```python
from build123d import *

# Parameters (mm, degrees)
CBORE_FOR_M3_HEX_SOCKET_HEAD_CAP_SCREW1_D           = 3.4
CBORE_FOR_M3_HEX_SOCKET_HEAD_CAP_SCREW1_CBORE_D     = 6.5
CBORE_FOR_M3_HEX_SOCKET_HEAD_CAP_SCREW1_CBORE_DEPTH = 3.4
F_20_0MM_DOWEL_HOLE1_D                              = 20


# Read off the part's stored shape, not the designer's step: M30 Machine Threads Stud1
with BuildPart() as part:
    # Sketch1 → Revolve1 (revolve)
    with BuildSketch(Plane.XY, mode=Mode.PRIVATE) as revolve1_sk:
        Polygon((0, 0), (41, 0), (41, 16), (6, 16), (6, 26), (0, 26), align=None)
    revolve(revolve1_sk.sketch.rotate(Axis((0, 0, 0), (1, 0, 0)), 90), axis=Axis((0, 0, 0), (1, 0, 0)))

    # M30 Machine Threads Stud1 outline → M30 Machine Threads Stud1 (revolve, cut)
    with BuildSketch(Plane.YX):
        Polygon((16, 41), (13.079, 41), (15, 39.079), (15, 26), (16, 26), align=None)
    revolve(axis=Axis((0, 0, 0), (1, 0, 0)), mode=Mode.SUBTRACT)

    # CBORE for M3 Hex Socket Head Cap Screw1 (through all)
    with Locations(Plane.ZY):
        with Locations((-21, 0), (0, 21), (21, 0), (0, -21)):
            CounterBoreHole(CBORE_FOR_M3_HEX_SOCKET_HEAD_CAP_SCREW1_D / 2, CBORE_FOR_M3_HEX_SOCKET_HEAD_CAP_SCREW1_CBORE_D / 2, CBORE_FOR_M3_HEX_SOCKET_HEAD_CAP_SCREW1_CBORE_DEPTH)

    # Ø20.0mm Dowel Hole1 (through all)
    with Locations(Plane.ZY):
        with Locations((0, 0)):
            Hole(F_20_0MM_DOWEL_HOLE1_D / 2)

    # Sketch9 → Cut-Revolve1 (revolve, cut)
    with BuildSketch(Plane.XY, mode=Mode.PRIVATE) as cut_revolve1_sk:
        Polygon((30, 15), (28.5, 13.5), (26, 13.5), (26, 15), align=None)
    revolve(cut_revolve1_sk.sketch.rotate(Axis((0, 0, 0), (1, 0, 0)), 90), axis=Axis((0, 0, 0), (1, 0, 0)), mode=Mode.SUBTRACT)


solid = part.part
```
Geometry check sheet. Reference: the model listing, model coordinates, mm. A direction names the side the tool comes from. Round coordinates to 2 decimals unless told otherwise and drop trailing zeros. Loops run counter-clockwise (first coordinate to the right, second up) from the corner with the lowest first, then second, coordinate; pieces in that order, holes last. Notation, with made-up numbers: (79.5, 76.25) - (127.5, 76.25) arc R32 cw to (127.5, 111.25) - close; hole circle Ø1 at (51.5, 23). An arc over 180 degrees is marked (long way). Write each question's results on one line, items separated by ' | '. Start each with the question number.
Q1. Gauge pin test, flat ends, axial feed: P1, Ø2, axis at y = 4, z = -20, coming from the +X side; P2, Ø6, axis at x = 13.5, y = -2, coming from the +Z side; P3, Ø4, axis at y = 21, z = 0, coming from the -X side; P4, Ø2, axis at y = 0, z = 21, coming from the -X side. Record the tip position at first contact, or that the pin passes through.
Q2. Thickness scan on line 1 (Y direction, x = 4, z = 0); line 2 (Y direction, x = 1.6, z = 0); line 3 (Y direction, x = 21, z = 0). Record the ranges inside material, lowest first. Write a range as [from, to].
Q3. Cross-section at C-C on y = 0. State how many separate pieces and enclosed holes the cut face has, and give its area (3 significant figures).
Q4. Release check for a two-part mould opening along X. For faces 1 (the flat face through (0, 0, 11)), 2 (the flat face through (26, 12, 7)), 3 (the cylindrical face through (4.72, -0.65, 19.43)), 4 (the cylindrical face through (27.23, 13.18, -2.93)) record: +X half, -X half, draft (parallel to the pull), parting line (faces both ways), or undercut.
Q5. Access from +Z, -Z, +X, -X, +Y, -Y to the whole of each face (thin tool, end or side, straight path). Record for faces 5 (the cylindrical face through (4.718, 22.686, 0.221)), 6 (the flat face through (3.4, -22.4, 1.4)), 7 (the cylindrical face through (34.476, -3.252, -14.643)).
Q6. Cross-section at A-A on z = -21. Enter the section's corners in (x, y), and give its area (3 significant figures).
Answers below:
1) P1: stops at x = 6 | P2: stops at z = 16 | P3: stops at x = 3.4 | P4: passes through
2) line 1: y = [-26, -22.7], [-19.3, -10], [10, 19.3], [22.7, 26] | line 2: y = [-26, -24.25], [-17.75, -10], [10, 17.75], [24.25, 26] | line 3: y = [-16, -10], [10, 16]
3) separate pieces: 4 | enclosed holes: 0 | area: 507 mm²
4) face 1: -X half | face 2: undercut | face 3: draft | face 4: undercut
5) face 5: +X, -X | face 6: -X | face 7: +X
6) outline: (0, -15.33) - (6, -15.33) - (6, -1.7) - (3.4, -1.7) - (3.4, -3.25) - (0, -3.25) - close; (0, 3.25) - (3.4, 3.25) - (3.4, 1.7) - (6, 1.7) - (6, 15.33) - (0, 15.33) - close | area: 153 mm²
